The listing builds one solid part. Answer for the finished solid, in the listing's coordinates (mm). Face numbers are marked on the shaded views. A direction names the side the tool comes from. Round coordinates to 2 decimals unless told otherwise and drop trailing zeros. Order: outer loops, then holes, each group sorted by start corner. A loop starts at its lowest first (then second) coordinate and runs counter-clockwise, first axis right, second up. Notation, with made-up numbers: (76, 50.5) -> (111, 50.5) arc R20 ccw to (111, 85.5) -> close; hole circle Ø8 at (66.25, -40). An arc over 180 degrees is marked (long way). Return JSON: item names as keys, results as strings. Group by question number.
(1) The part is cut by section A-A (y = 1.25). Determine the outline of the cut face in (x, z).
(2) Which of the six approach directions +Z, -Z, +X, -X, +Y, -Y give full straight-line access (tool end or side, diameter ignored) to the marked faces 4, 5, 6 and 7?
(3) Determine the mould class of the marked faces 1, 2 and 3 for opening direction X: +X half, -X half, draft (parallel to the pull), parting line (faces both ways), or undercut.
(4) Consider line 1 (Z direction, x = 0, y = -0.5); line 2 (Z direction, x = 0, y = 1.25); line 3 (Z direction, x = 4.75, y = -4). Determine where each line is inside the solid, lowest interval first. Write a range as [from, to].
(5) The part is cut by section D-D (y = -0.5). Determine the outline of the cut face in (x, z).
(6) The part is cut by section B-B (x = 0). Determine the outline of the cut face in (y, z), plus the area to 3 significant figures.
(7) Each of these flat-tipped pins is pushed along its axis until it touches: pin 1 (3 mm diameter, centred on x = -3.5, z = 10, fed in from +Y); pin 2 (4.5 mm diameter, centred on x = 0, z = 13, fed in from -Y); pin 3 (2.5 mm diameter, centred on x = 0, z = 5, fed in from +Y); pin 4 (3 mm diameter, centred on y = -4, z = 5.5, fed in from -X). Where does it stop, or does it pass through?
(8) The part is cut by section C-C (z = 5). Determine the outline of the cut face in (x, y).
from build123d import *

# Parameters (mm, degrees)
SKETCH_1_W          = 7.7
SKETCH_1_H          = 7.7
EXTRUDE_1_DEPTH     = 21
SKETCH_2_W          = 11.7
SKETCH_2_H          = 11.7
EXTRUDE_2_DEPTH     = 2
CHAMFER_1_SIZE      = 3
FILLET_2_R          = 1
SKETCH_5_R          = 1.65
CUT_EXTRUDE_2_DEPTH = 24


with BuildPart() as part:
    # 草图1 → 凸台-拉伸1 (new body)
    with BuildSketch(Plane.XY):
        Rectangle(SKETCH_1_W, SKETCH_1_H)
    extrude(amount=EXTRUDE_1_DEPTH)

    # 草图2 → 凸台-拉伸2 (add)
    with BuildSketch(Plane(origin=(0, 0, 0), x_dir=(-1, 0, 0), z_dir=(0, 0, -1))):
        Rectangle(SKETCH_2_W, SKETCH_2_H)
    extrude(amount=EXTRUDE_2_DEPTH)

    # 倒角1
    chamfer_1_edges = [part.edges().sort_by_distance(p)[0] for p in [
        (-3.85, 0, 21),
        (0, -3.85, 21),
        (3.85, 0, 21),
        (0, 3.85, 21),
    ]]
    chamfer(chamfer_1_edges, length=CHAMFER_1_SIZE)

    # 圆角2
    fillet_2_edges = [part.edges().sort_by_distance(p)[0] for p in [
        (-5.85, -5.85, -1),
        (-5.85, 5.85, -1),
        (5.85, 5.85, -1),
        (5.85, -5.85, -1),
        (-3.85, -3.85, 9),
        (-3.85, 3.85, 9),
        (3.85, -3.85, 9),
        (3.85, 3.85, 9),
    ]]
    fillet(fillet_2_edges, radius=FILLET_2_R)

    # 草图5 → 切除-拉伸2 (cut)
    with BuildSketch(Plane.XZ.offset(3.85)):
        with Locations((0, 5)):
            Circle(SKETCH_5_R)
        with Locations((0, 13)):
            Circle(SKETCH_5_R)
    extrude(amount=-CUT_EXTRUDE_2_DEPTH, mode=Mode.SUBTRACT)


solid = part.part
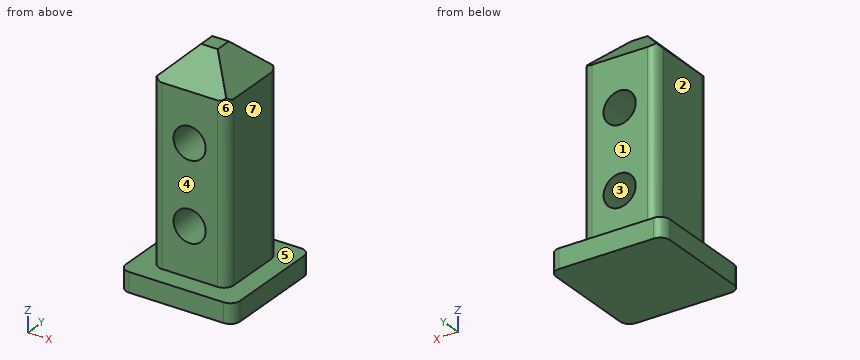
Answer below:
{
 "1": {"outline": "(-5.85, -2) -> (5.85, -2) -> (5.85, 0) -> (3.85, 0) -> (3.85, 18) -> (1.25, 20.6) -> (-1.25, 20.6) -> (-3.85, 18) -> (-3.85, 0) -> (-5.85, 0) -> close; hole circle Ø3.3 at (0, 5); hole circle Ø3.3 at (0, 13)"},
 "2": {"face 4": "+Z, +X, -X, -Y", "face 5": "+Z", "face 6": "+Z, +X, -Y", "face 7": "+Z, +X, +Y, -Y"},
 "3": {"face 1": "draft", "face 2": "-X half", "face 3": "undercut"},
 "4": {"line 1": "z = [-2, 3.35], [6.65, 11.35], [14.65, 21]", "line 2": "z = [-2, 3.35], [6.65, 11.35], [14.65, 20.6]", "line 3": "z = [-2, 0]"},
 "5": {"outline": "(-5.85, -2) -> (5.85, -2) -> (5.85, 0) -> (3.85, 0) -> (3.85, 18) -> (0.85, 21) -> (-0.85, 21) -> (-3.85, 18) -> (-3.85, 0) -> (-5.85, 0) -> close; hole circle Ø3.3 at (0, 5); hole circle Ø3.3 at (0, 13)"},
 "6": {"outline": "(-5.85, -2) -> (5.85, -2) -> (5.85, 0) -> (3.85, 0) -> (3.85, 3.35) -> (-3.85, 3.35) -> (-3.85, 0) -> (-5.85, 0) -> close; (-3.85, 6.65) -> (3.85, 6.65) -> (3.85, 11.35) -> (-3.85, 11.35) -> close; (-3.85, 14.65) -> (3.85, 14.65) -> (3.85, 18) -> (0.85, 21) -> (-0.85, 21) -> (-3.85, 18) -> close", "area": "125 mm²"},
 "7": {"pin 1": "stops at y = 3.85", "pin 2": "stops at y = -3.85", "pin 3": "passes through", "pin 4": "stops at x = -3.85"},
 "8": {"outline": "(-3.85, -2.85) arc R1 ccw to (-2.85, -3.85) -> (-1.65, -3.85) -> (-1.65, 3.85) -> (-2.85, 3.85) arc R1 ccw to (-3.85, 2.85) -> close; (1.65, -3.85) -> (2.85, -3.85) arc R1 ccw to (3.85, -2.85) -> (3.85, 2.85) arc R1 ccw to (2.85, 3.85) -> (1.65, 3.85) -> close"}
}
